Verification items for this drawing (mm, ordinates from the low corner). Coordinates: 2 decimals unless noted, no trailing zeros. Order: outer loops, then holes, each group sorted by start corner. A loop starts at its lowest first (then second) coordinate and runs counter-clockwise, first axis right, second up. Notation, with made-up numbers: (80, 53.5) - (100, 53.5) arc R22 ccw to (100, 61.5) - close; hole circle Ø7 at (43, 45). An arc over 180 degrees is marked (long way). Use CSV: the item, a comma, the result in double quotes. Start each with the question number.
1) Thickness scan on probe 1 along X at (y, z) = (1.9, 135); probe 2 along Z at (x, y) = (222, 1.85) (1 decimal); probe 3 along Z at (x, y) = (250, 2.25). Record the ranges inside material, lowest first. Write a range as [from, to].
2) Depth check by flat-ended pin: P1, Ø21.5, axis at x = 135, z = 250, coming from the +Y side; P2, Ø2, axis at y = 2, z = 230.5, coming from the +X side; P3, Ø1.5, axis at x = 48, y = 1, coming from the +Z side (1 decimal). Enter the tip coordinate at first touch or a pass-through.
3) Sectioned sample at B-B, the plane x = 135. Record the cut outline in (y, z).
4) Sectioned sample at C-C, the plane y = 3.65. Count the separate pieces of the cut face and the enclosed holes in it, and give its area (3 significant figures).
5) Sectioned sample at D-D, the plane x = 64. Record the cut outline in (y, z) (1 decimal), and give its area (3 significant figures).
6) Sectioned sample at A-A, the plane z = 135. Record the cut outline in (x, y), and give its area (3 significant figures).
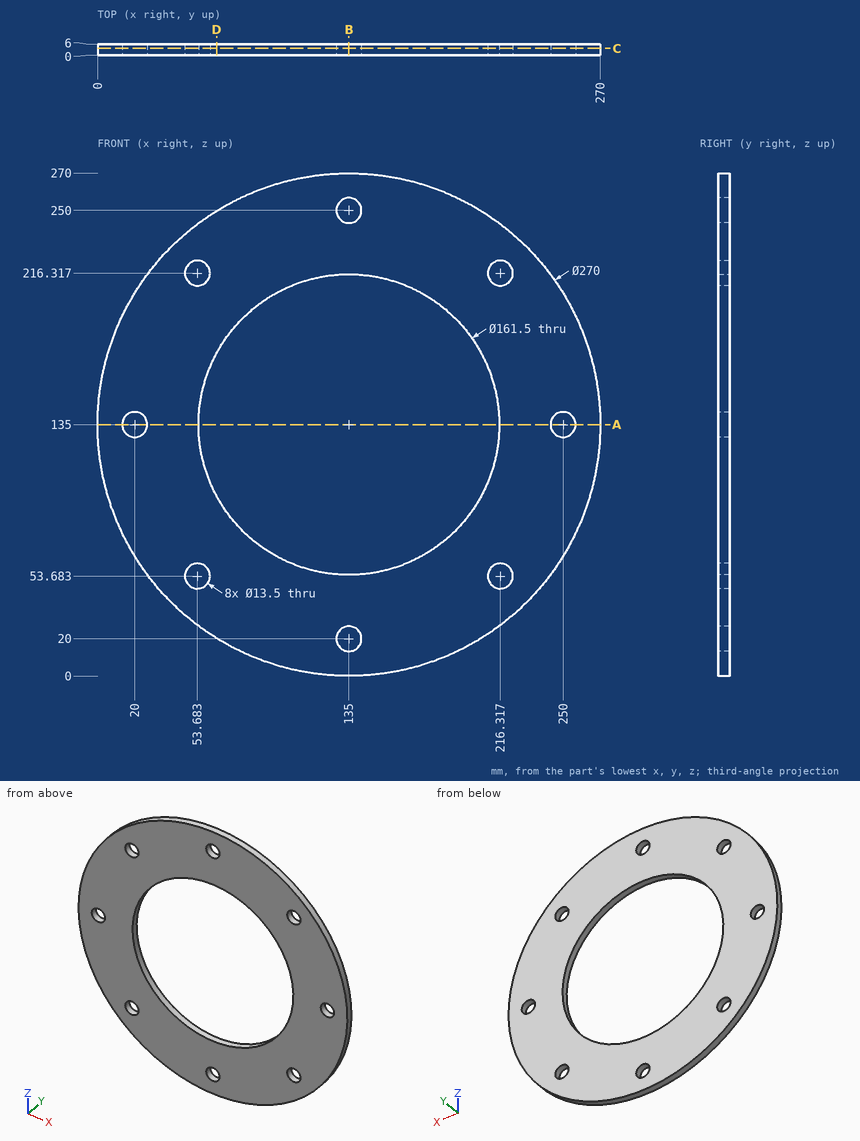
Evaluation:
1,probe 1,"[0, 13.25], [26.75, 54.25], [215.75, 243.25], [256.75, 270]"
1,probe 2,"[31.8, 50], [57.3, 212.7], [220, 238.2]"
1,probe 3,"[64.29, 128.25], [141.75, 205.71]"
2,P1,"y = 6"
2,P2,"x = 231.41"
2,P3,"z = 238.9"
3,outline,"(0, 0) - (6, 0) - (6, 13.25) - (0, 13.25) - close; (0, 26.75) - (6, 26.75) - (6, 54.25) - (0, 54.25) - close; (0, 215.75) - (6, 215.75) - (6, 243.25) - (0, 243.25) - close; (0, 256.75) - (6, 256.75) - (6, 270) - (0, 270) - close"
4,separate pieces,"1"
4,enclosed holes,"9"
4,area,"35,600 mm²"
5,outline,"(0, 20.2) - (6, 20.2) - (6, 96.5) - (0, 96.5) - close; (0, 173.5) - (6, 173.5) - (6, 249.8) - (0, 249.8) - close"
5,area,"916 mm²"
6,outline,"(0, 0) - (13.25, 0) - (13.25, 6) - (0, 6) - close; (26.75, 0) - (54.25, 0) - (54.25, 6) - (26.75, 6) - close; (215.75, 0) - (243.25, 0) - (243.25, 6) - (215.75, 6) - close; (256.75, 0) - (270, 0) - (270, 6) - (256.75, 6) - close"
6,area,"489 mm²"
